The drawing under review shows one solid part. Ordinate dimensions are in mm from its lowest x, y, z. Coordinates: 2 decimals unless noted, no trailing zeros. Write each loop counter-clockwise with the first axis right and the second up, starting at its lowest first coordinate (ties: lowest second). Pieces come first, ordered by that corner, then holes. Notation, with made-up numbers: (81.25, 53) -> (89.25, 53) arc R11 ccw to (89.25, 58) -> close; hole circle Ø4 at (28.25, 17.5). An arc over 180 degrees is marked (long way). One line per question, with ' | ' between items. Start each with the question number.
Q1. For P1, Ø1, axis at x = 57, y = 0.5, coming from the -Z side; P2, Ø1, axis at x = 57.5, y = 1, coming from the +Z side, all flat-tipped, find the tip position at first contact; note any pin that passes through.
Q2. Wall thickness on probe 1 along Z at (x, y) = (30.5, 1.95); probe 2 along Y at (x, z) = (15.5, 35); probe 3 along X at (y, z) = (1.45, 10): over which ranges is each line inside the solid? List them lowest first.
Q3. Add section D-D on z = 16.5. State the section outline as (x, y) points.
Q4. Draft analysis for pull direction Z (two halves, no side actions). For the marked faces 1 and 2, state which applies: pulls with the +Z half, pulls with the -Z half, needs draft (parallel to the pull), parting line crosses it, or undercut.
Q5. Add section A-A on z = 25. Give the number of separate pieces and of enclosed holes in the cut face.
Q6. Add section B-B on x = 30.15. State the section outline as (y, z) points.
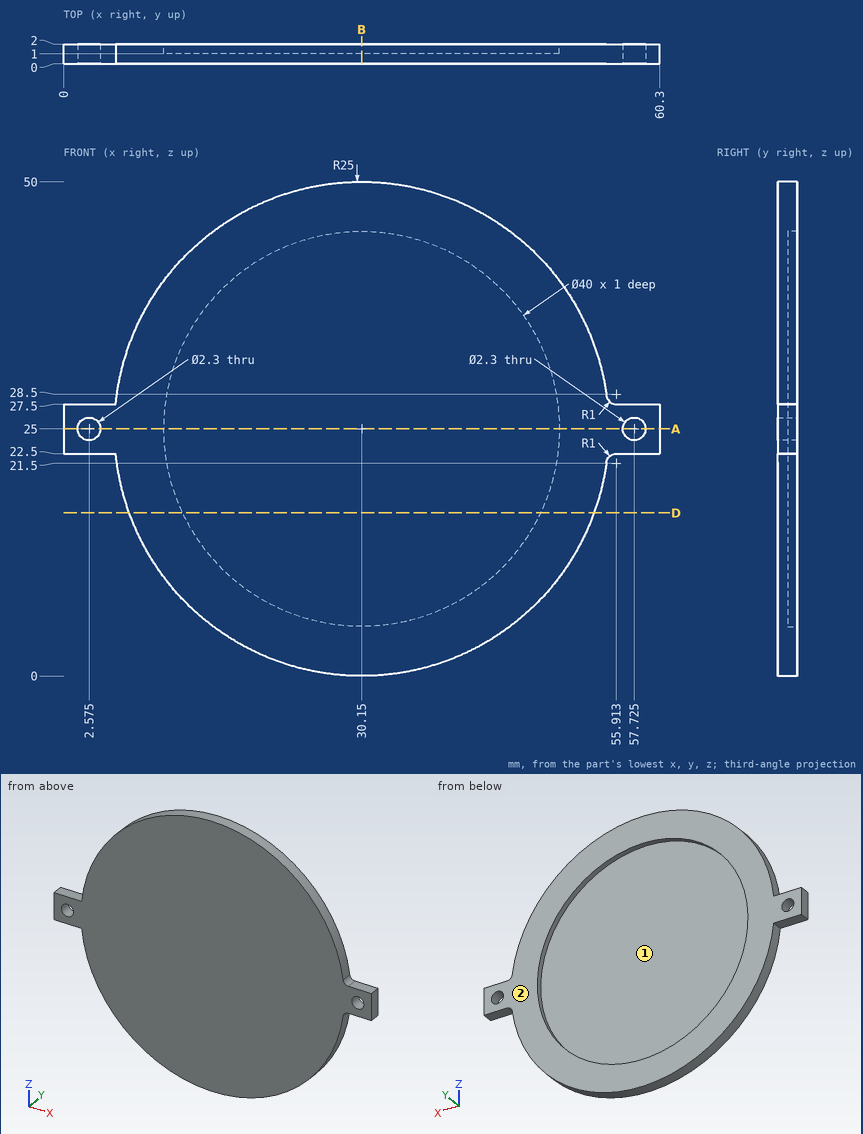
Output values:
1) P1: stops at z = 22.5 | P2: stops at z = 27.5
2) probe 1: z = 0 to 5, 45 to 50 | probe 2: y = 0 to 1 | probe 3: x = 10.15 to 16.92, 43.38 to 50.15
3) outline: (6.64, 0) -> (53.66, 0) -> (53.66, 2) -> (48.25, 2) -> (48.25, 1) -> (12.05, 1) -> (12.05, 2) -> (6.64, 2) -> close
4) face 1: undercut | face 2: needs draft
5) separate pieces: 3 | enclosed holes: 0
6) outline: (0, 0) -> (2, 0) -> (2, 5) -> (1, 5) -> (1, 45) -> (2, 45) -> (2, 50) -> (0, 50) -> close
